The model under review builds one solid part; all positions refer to its coordinate system, in mm. Give positions to 0.01 mm unless a question says otherwise; leave off trailing zeros. Order: outer loops, then holes, each group sorted by start corner. A loop starts at its lowest first (then second) coordinate and runs counter-clockwise, first axis right, second up.
```python
from build123d import *

# Parameters (mm, degrees)
SKETCH1_R               = 14.28115
SKETCH1_R_2             = 19.177
BOSS_EXTRUDE1_DEPTH     = 3.175
F_10_CLEARANCE_HOLE1_D  = 5.1054
F_1_4_CLEARANCE_HOLE1_D = 6.7564
SKETCH6_R               = 2.5527
CUT_EXTRUDE1_DEPTH      = 4.175
FILLET1_R               = 7.62
CUT_EXTRUDE2_DEPTH      = 4.175
FILLET2_R               = 9.525


with BuildPart() as part:
    # Sketch1 → Boss-Extrude1 (new body)
    with BuildSketch(Plane(origin=(0, 0, 0), x_dir=(1, 0, 0), z_dir=(0, 1, 0))):
        with BuildLine():
            Line((85.884602434, 50.671947857), (-3.15409287, 44.337954375))
            ThreePointArc((-3.15409287, 44.337954375), (-44.45, 0), (-3.15409287, -44.337954375))
            Line((-3.15409287, -44.337954375), (85.884602434, -50.671947857))
            ThreePointArc((85.884602434, -50.671947857), (140.28928, 0), (85.884602434, 50.671947857))
        make_face()
        with Locations((89.48928, 0)):
            Circle(SKETCH1_R, mode=Mode.SUBTRACT)
        Circle(SKETCH1_R_2, mode=Mode.SUBTRACT)
    extrude(amount=BOSS_EXTRUDE1_DEPTH)

    # #10 Clearance Hole1 (through all)
    with Locations(Plane(origin=(0, 3.175, 0), x_dir=(1, 0, 0), z_dir=(0, 1, 0))):
        with Locations((-17.960512242, 17.960512242), (17.960512242, 17.960512242), (17.960512242, -17.960512242), (-17.960512242, -17.960512242), (-31.8135, 0), (34.925, 34.314713318), (34.925, -34.314713318)):
            Hole(F_10_CLEARANCE_HOLE1_D / 2)

    # 1/4 Clearance Hole1 (through all)
    with Locations(Plane(origin=(0, 3.175, 0), x_dir=(1, 0, 0), z_dir=(0, 1, 0))):
        with Locations((54.56428, 34.925), (54.56428, -34.925), (114.88928, 25.4), (114.88928, -25.4)):
            Hole(F_1_4_CLEARANCE_HOLE1_D / 2)

    # Sketch6 → Cut-Extrude1 (cut, through all)
    with BuildSketch(Plane(origin=(0, 3.175, 0), x_dir=(1, 0, 0), z_dir=(0, 1, 0))):
        with BuildLine():
            Line((-9.48365621, 16.667861107), (-14.368409794, 21.552614691))
            ThreePointArc((-14.368409794, 21.552614691), (-21.552614691, 21.552614691), (-21.552614691, 14.368409794))
            Line((-21.552614691, 14.368409794), (-16.667861107, 9.48365621))
            ThreePointArc((-16.667861107, 9.48365621), (-13.560186743, 13.560186743), (-9.48365621, 16.667861107))
        make_face()
        with Locations((-17.960512242, 17.960512242)):
            Circle(SKETCH6_R, mode=Mode.SUBTRACT)
        with BuildLine():
            ThreePointArc((16.667861107, -9.48365621), (13.560186743, -13.560186743), (9.48365621, -16.667861107))
            Line((9.48365621, -16.667861107), (14.368409794, -21.552614691))
            ThreePointArc((14.368409794, -21.552614691), (21.552614691, -21.552614691), (21.552614691, -14.368409794))
            Line((21.552614691, -14.368409794), (16.667861107, -9.48365621))
        make_face()
        with Locations((17.960512242, -17.960512242)):
            Circle(SKETCH6_R, mode=Mode.SUBTRACT)
    extrude(amount=-CUT_EXTRUDE1_DEPTH, mode=Mode.SUBTRACT)

    # Fillet1
    fillet1_edges = [part.edges().sort_by_distance(p)[0] for p in [
        (9.48365621, 1.5875, 16.667861107),
        (16.667861107, 1.5875, 9.48365621),
        (-9.48365621, 1.5875, -16.667861107),
        (-16.667861107, 1.5875, -9.48365621),
    ]]
    fillet(fillet1_edges, radius=FILLET1_R)

    # Sketch7 → Cut-Extrude2 (cut, through all)
    with BuildSketch(Plane(origin=(0, 3.175, 0), x_dir=(1, 0, 0), z_dir=(0, 1, 0))):
        Polygon((43.815, 47.679219957), (43.815, -47.679219957), (-626.42496, 0), align=None)
    extrude(amount=-CUT_EXTRUDE2_DEPTH, mode=Mode.SUBTRACT)

    # Fillet2
    fillet2_edges = [part.edges().sort_by_distance(p)[0] for p in [
        (43.815, 1.5875, 47.679219957),
        (43.815, 1.5875, -47.679219957),
    ]]
    fillet(fillet2_edges, radius=FILLET2_R)


solid = part.part
```
Item 1: Take a section at A-A (z = 0). Give the boundary of the cut face in (x, y) (3 decimals).
Values found:
outline: (43.815, 0) - (75.208, 0) - (75.208, 3.175) - (43.815, 3.175) - close; (103.77, 0) - (140.289, 0) - (140.289, 3.175) - (103.77, 3.175) - close
Item 2: Take a section at D-D (z = -16.5). Give the boundary of the cut face in (x, y) (3 decimals).
Values found:
outline: (43.815, 0) - (137.535, 0) - (137.535, 3.175) - (43.815, 3.175) - close
Item 3: For line 1 (Z direction, x = 52.5, y = 2.7); line 2 (Z direction, x = 89.5, y = 0.25); line 3 (X direction, y = 2.75, z = -5) (3 decimals), list the stretches that pass through material, from the lowest coordinate up.
Values found:
line 1: z = -48.3 to -37.6, -32.25 to 32.25, 37.6 to 48.3
line 2: z = -50.8 to -14.28, 14.28 to 50.8
line 3: x = 43.815 to 76.112, 102.867 to 140.043
Item 4: Clearance check with flat-ended pins moving along their axes: pin 1 Ø4 at (x, z) = (54.56, 34.92) entering from -Y; pin 2 Ø6 at (x, z) = (66, -19) entering from -Y; pin 3 Ø1 at (y, z) = (2.5, 11) entering from +X. State where each tip first meets the part, or that it passes through.
Values found:
pin 1: passes through
pin 2: stops at y = 0
pin 3: stops at x = 139.19
Item 5: Take a section at B-B (y = 2.6). Give the boundary of the cut face in (x, z) (3 decimals).
Values found:
outline: (43.815, -38.808) arc R9.525 ccw to (52.664, -48.309) - (85.885, -50.672) arc R50.8 ccw (long way) to (85.885, 50.672) - (52.664, 48.309) arc R9.525 ccw to (43.815, 38.808) - close; hole circle Ø6.756 at (54.564, -34.925); hole circle Ø6.756 at (54.564, 34.925); hole circle Ø28.562 at (89.489, 0); hole circle Ø6.756 at (114.889, -25.4); hole circle Ø6.756 at (114.889, 25.4)
Item 6: Take a section at C-C (x = 91). Give the boundary of the cut face in (y, z) (3 decimals), and give its area (3 significant figures).
Values found:
outline: (0, -50.778) - (3.175, -50.778) - (3.175, -14.201) - (0, -14.201) - close; (0, 14.201) - (3.175, 14.201) - (3.175, 50.778) - (0, 50.778) - close
area: 232 mm2
Item 7: Draft analysis for pull direction X (two halves, no side actions). For faces 1 (the cylindrical face through (102.68, 1.57, 5.47)), 2 (the flat face through (43.815, 2, -1)), 3 (the flat face through (81, 0, -12)), state which applies: released by +X, released by -X, zero draft, split by the parting line, or undercut.
Values found:
face 1: undercut
face 2: released by -X
face 3: zero draft
